Design review of the part built by this model. Coordinates are the model's own, in mm. Face numbers are marked on the shaded views. A direction names the side the tool comes from. Round coordinates to 2 decimals unless told otherwise and drop trailing zeros. Loops run counter-clockwise (first coordinate to the right, second up) from the corner with the lowest first, then second, coordinate; pieces in that order, holes last. Notation, with made-up numbers: (47.5, 45.25) - (62.5, 45.25) arc R22 ccw to (62.5, 75.25) - close; hole circle Ø3 at (48.5, 54.5). An arc over 180 degrees is marked (long way). Return JSON: item names as keys, results as strings. Group by question number.
(1) Wall thickness on L1, parallel to Y at x = -15.5, z = -20.85; L2, parallel to X at y = -25.75, z = 38.5; L3, parallel to Z at x = -5.5, y = 34.5: over which ranges is each line inside the solid? List them lowest first. Write a range as [from, to].
(2) We need section B-B, the plane y = 37. Write out the cut boundary in (x, z).
(3) Clearance check with flat-ended pins moving along their axes: pin 1 (1.5 mm diameter, centred on x = -6.5, z = 6, fed in from -Y); pin 2 (21.5 mm diameter, centred on x = -3, z = 15, fed in from +Y); pin 3 (6.5 mm diameter, centred on y = -36.5, z = 38.5, fed in from -X). State where each tip first meets the part, or that it passes through.
(4) We need section A-A, the plane x = -15.5. Write out the cut boundary in (y, z).
(5) For the marked faces 1, 2, 3, 4 and 5, list the 3-axis set-ups (+Z, -Z, +X, -X, +Y, -Y) from which the entire face can be reached by the end or side of a thin tool; tool diameter is ignored.
(6) We need section C-C, the plane y = 26. Write out the cut boundary in (x, z), and give its area (3 significant figures).
(7) We need section D-D, the plane z = 31.5. Write out the cut boundary in (x, y), and give its area (3 significant figures).
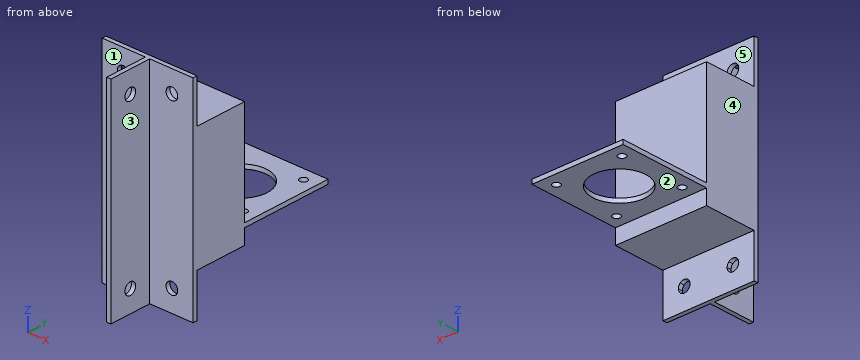
from build123d import *

# Parameters (mm, degrees)
SKETCH1_W           = 43
SKETCH1_H           = 2
BOSS_EXTRUDE1_DEPTH = 43
SKETCH1_3_W         = 43
SKETCH1_3_H         = 97
BOSS_EXTRUDE2_DEPTH = 26.5
CUT_EXTRUDE1_REACH  = 85.278
SKETCH2_R           = 12.5
SKETCH2_R_2         = 1.75
CUT_EXTRUDE2_REACH  = 70.29
SKETCH1_4_R         = 2.75
SKETCH3_W           = 43
SKETCH3_H           = 20
CUT_EXTRUDE3_DEPTH  = 24.5
SKETCH4_W           = 2
SKETCH4_H           = 97
BOSS_EXTRUDE3_DEPTH = 20
CUT_EXTRUDE4_REACH  = 72.857
SKETCH5_R           = 2.75


with BuildPart() as part:
    # Sketch1 → Boss-Extrude1 (new body)
    with BuildSketch(Plane(origin=(0, 0, 0), x_dir=(1, 0, 0), z_dir=(0, 1, 0))):
        with Locations((0, 20.5)):
            Rectangle(SKETCH1_W, SKETCH1_H)
    extrude(amount=BOSS_EXTRUDE1_DEPTH)

    # Sketch1_3 → Boss-Extrude2 (add)
    with BuildSketch(Plane(origin=(0, 0, 0), x_dir=(1, 0, 0), z_dir=(0, 1, 0))):
        Rectangle(SKETCH1_3_W, SKETCH1_3_H)
    extrude(amount=-BOSS_EXTRUDE2_DEPTH)

    # Sketch2 → Cut-Extrude1 (cut, up to next)
    with BuildSketch(Plane.XY.offset(-19.5), mode=Mode.PRIVATE) as cut_extrude1_sk1:
        with Locations((0, 21.5)):
            Circle(SKETCH2_R)
    cut_extrude1_tool1 = extrude(cut_extrude1_sk1.sketch, amount=-CUT_EXTRUDE1_REACH, mode=Mode.PRIVATE) & part.part
    # Sketch2 → Cut-Extrude1 (cut, up to next)
    with BuildSketch(Plane.XY.offset(-19.5), mode=Mode.PRIVATE) as cut_extrude1_sk2:
        with Locations((-15.5, 37)):
            Circle(SKETCH2_R_2)
    cut_extrude1_tool2 = extrude(cut_extrude1_sk2.sketch, amount=-CUT_EXTRUDE1_REACH, mode=Mode.PRIVATE) & part.part
    # Sketch2 → Cut-Extrude1 (cut, up to next)
    with BuildSketch(Plane.XY.offset(-19.5), mode=Mode.PRIVATE) as cut_extrude1_sk3:
        with Locations((15.5, 37)):
            Circle(SKETCH2_R_2)
    cut_extrude1_tool3 = extrude(cut_extrude1_sk3.sketch, amount=-CUT_EXTRUDE1_REACH, mode=Mode.PRIVATE) & part.part
    # Sketch2 → Cut-Extrude1 (cut, up to next)
    with BuildSketch(Plane.XY.offset(-19.5), mode=Mode.PRIVATE) as cut_extrude1_sk4:
        with Locations((15.5, 6)):
            Circle(SKETCH2_R_2)
    cut_extrude1_tool4 = extrude(cut_extrude1_sk4.sketch, amount=-CUT_EXTRUDE1_REACH, mode=Mode.PRIVATE) & part.part
    # Sketch2 → Cut-Extrude1 (cut, up to next)
    with BuildSketch(Plane.XY.offset(-19.5), mode=Mode.PRIVATE) as cut_extrude1_sk5:
        with Locations((-15.5, 6)):
            Circle(SKETCH2_R_2)
    cut_extrude1_tool5 = extrude(cut_extrude1_sk5.sketch, amount=-CUT_EXTRUDE1_REACH, mode=Mode.PRIVATE) & part.part
    add(cut_extrude1_tool1.solids().sort_by_distance((0, 21.5, -19.5))[0], mode=Mode.SUBTRACT)
    add(cut_extrude1_tool2.solids().sort_by_distance((-15.5, 37, -19.5))[0], mode=Mode.SUBTRACT)
    add(cut_extrude1_tool3.solids().sort_by_distance((15.5, 37, -19.5))[0], mode=Mode.SUBTRACT)
    add(cut_extrude1_tool4.solids().sort_by_distance((15.5, 6, -19.5))[0], mode=Mode.SUBTRACT)
    add(cut_extrude1_tool5.solids().sort_by_distance((-15.5, 6, -19.5))[0], mode=Mode.SUBTRACT)

    # Sketch1_4 → Cut-Extrude2 (cut, up to next)
    with BuildSketch(Plane(origin=(0, 0, 0), x_dir=(1, 0, 0), z_dir=(0, 1, 0)), mode=Mode.PRIVATE) as cut_extrude2_sk1:
        with Locations(Location((-11.5, -38.5, 0), (0, 0, 270))):
            Circle(SKETCH1_4_R)
    cut_extrude2_tool1 = extrude(cut_extrude2_sk1.sketch, amount=-CUT_EXTRUDE2_REACH, mode=Mode.PRIVATE) & part.part
    # Sketch1_4 → Cut-Extrude2 (cut, up to next)
    with BuildSketch(Plane(origin=(0, 0, 0), x_dir=(1, 0, 0), z_dir=(0, 1, 0)), mode=Mode.PRIVATE) as cut_extrude2_sk2:
        with Locations(Location((11.5, -38.5, 0), (0, 0, 270))):
            Circle(SKETCH1_4_R)
    cut_extrude2_tool2 = extrude(cut_extrude2_sk2.sketch, amount=-CUT_EXTRUDE2_REACH, mode=Mode.PRIVATE) & part.part
    # Sketch1_4 → Cut-Extrude2 (cut, up to next)
    with BuildSketch(Plane(origin=(0, 0, 0), x_dir=(1, 0, 0), z_dir=(0, 1, 0)), mode=Mode.PRIVATE) as cut_extrude2_sk3:
        with BuildLine():
            ThreePointArc((-8.75, 38.5), (-12.589033706, 41.025174368), (-13.387458609, 36.5))
            Line((-13.387458609, 36.5), (-9.612541391, 36.5))
            ThreePointArc((-9.612541391, 36.5), (-8.974825632, 37.410966294), (-8.75, 38.5))
        make_face()
    cut_extrude2_tool3 = extrude(cut_extrude2_sk3.sketch, amount=-CUT_EXTRUDE2_REACH, mode=Mode.PRIVATE) & part.part
    # Sketch1_4 → Cut-Extrude2 (cut, up to next)
    with BuildSketch(Plane(origin=(0, 0, 0), x_dir=(1, 0, 0), z_dir=(0, 1, 0)), mode=Mode.PRIVATE) as cut_extrude2_sk4:
        with BuildLine():
            Line((-9.612541391, 36.5), (-13.387458609, 36.5))
            ThreePointArc((-13.387458609, 36.5), (-11.5, 35.75), (-9.612541391, 36.5))
        make_face()
    cut_extrude2_tool4 = extrude(cut_extrude2_sk4.sketch, amount=-CUT_EXTRUDE2_REACH, mode=Mode.PRIVATE) & part.part
    # Sketch1_4 → Cut-Extrude2 (cut, up to next)
    with BuildSketch(Plane(origin=(0, 0, 0), x_dir=(1, 0, 0), z_dir=(0, 1, 0)), mode=Mode.PRIVATE) as cut_extrude2_sk5:
        with BuildLine():
            ThreePointArc((9.612541391, 36.5), (11.5, 35.75), (13.387458609, 36.5))
            Line((13.387458609, 36.5), (9.612541391, 36.5))
        make_face()
    cut_extrude2_tool5 = extrude(cut_extrude2_sk5.sketch, amount=-CUT_EXTRUDE2_REACH, mode=Mode.PRIVATE) & part.part
    # Sketch1_4 → Cut-Extrude2 (cut, up to next)
    with BuildSketch(Plane(origin=(0, 0, 0), x_dir=(1, 0, 0), z_dir=(0, 1, 0)), mode=Mode.PRIVATE) as cut_extrude2_sk6:
        with BuildLine():
            Line((9.612541391, 36.5), (13.387458609, 36.5))
            ThreePointArc((13.387458609, 36.5), (14.025174368, 37.410966294), (14.25, 38.5))
            ThreePointArc((14.25, 38.5), (10.410966294, 41.025174368), (9.612541391, 36.5))
        make_face()
    cut_extrude2_tool6 = extrude(cut_extrude2_sk6.sketch, amount=-CUT_EXTRUDE2_REACH, mode=Mode.PRIVATE) & part.part
    # Sketch1_4 → Cut-Extrude2 (cut, up to next)
    with BuildSketch(Plane(origin=(0, 0, 0), x_dir=(1, 0, 0), z_dir=(0, 1, 0)), mode=Mode.PRIVATE) as cut_extrude2_sk7:
        with BuildLine():
            ThreePointArc((9.612541391, 36.5), (11.5, 35.75), (13.387458609, 36.5))
            Line((13.387458609, 36.5), (9.612541391, 36.5))
        make_face()
    cut_extrude2_tool7 = extrude(cut_extrude2_sk7.sketch, amount=-CUT_EXTRUDE2_REACH, mode=Mode.PRIVATE) & part.part
    # Sketch1_4 → Cut-Extrude2 (cut, up to next)
    with BuildSketch(Plane(origin=(0, 0, 0), x_dir=(1, 0, 0), z_dir=(0, 1, 0)), mode=Mode.PRIVATE) as cut_extrude2_sk8:
        with BuildLine():
            Line((9.612541391, 36.5), (13.387458609, 36.5))
            ThreePointArc((13.387458609, 36.5), (14.025174368, 37.410966294), (14.25, 38.5))
            ThreePointArc((14.25, 38.5), (10.410966294, 41.025174368), (9.612541391, 36.5))
        make_face()
    cut_extrude2_tool8 = extrude(cut_extrude2_sk8.sketch, amount=-CUT_EXTRUDE2_REACH, mode=Mode.PRIVATE) & part.part
    # Sketch1_4 → Cut-Extrude2 (cut, up to next)
    with BuildSketch(Plane(origin=(0, 0, 0), x_dir=(1, 0, 0), z_dir=(0, 1, 0)), mode=Mode.PRIVATE) as cut_extrude2_sk9:
        with BuildLine():
            ThreePointArc((-8.75, 38.5), (-12.589033706, 41.025174368), (-13.387458609, 36.5))
            Line((-13.387458609, 36.5), (-9.612541391, 36.5))
            ThreePointArc((-9.612541391, 36.5), (-8.974825632, 37.410966294), (-8.75, 38.5))
        make_face()
    cut_extrude2_tool9 = extrude(cut_extrude2_sk9.sketch, amount=-CUT_EXTRUDE2_REACH, mode=Mode.PRIVATE) & part.part
    # Sketch1_4 → Cut-Extrude2 (cut, up to next)
    with BuildSketch(Plane(origin=(0, 0, 0), x_dir=(1, 0, 0), z_dir=(0, 1, 0)), mode=Mode.PRIVATE) as cut_extrude2_sk10:
        with BuildLine():
            Line((-9.612541391, 36.5), (-13.387458609, 36.5))
            ThreePointArc((-13.387458609, 36.5), (-11.5, 35.75), (-9.612541391, 36.5))
        make_face()
    cut_extrude2_tool10 = extrude(cut_extrude2_sk10.sketch, amount=-CUT_EXTRUDE2_REACH, mode=Mode.PRIVATE) & part.part
    add(cut_extrude2_tool1.solids().sort_by_distance((-11.5, 0, 38.5))[0], mode=Mode.SUBTRACT)
    add(cut_extrude2_tool2.solids().sort_by_distance((11.5, 0, 38.5))[0], mode=Mode.SUBTRACT)
    add(cut_extrude2_tool3.solids().sort_by_distance((-11.5, 0, -38.705511))[0], mode=Mode.SUBTRACT)
    add(cut_extrude2_tool4.solids().sort_by_distance((-11.5, 0, -36.196191))[0], mode=Mode.SUBTRACT)
    add(cut_extrude2_tool5.solids().sort_by_distance((11.5, 0, -36.196191))[0], mode=Mode.SUBTRACT)
    add(cut_extrude2_tool6.solids().sort_by_distance((11.5, 0, -38.705511))[0], mode=Mode.SUBTRACT)
    add(cut_extrude2_tool7.solids().sort_by_distance((11.5, 0, -36.196191))[0], mode=Mode.SUBTRACT)
    add(cut_extrude2_tool8.solids().sort_by_distance((11.5, 0, -38.705511))[0], mode=Mode.SUBTRACT)
    add(cut_extrude2_tool9.solids().sort_by_distance((-11.5, 0, -38.705511))[0], mode=Mode.SUBTRACT)
    add(cut_extrude2_tool10.solids().sort_by_distance((-11.5, 0, -36.196191))[0], mode=Mode.SUBTRACT)

    # Sketch3 → Cut-Extrude3 (cut)
    with BuildSketch(Plane(origin=(0, 0, 0), x_dir=(1, 0, 0), z_dir=(0, 1, 0))):
        with Locations((0, -38.5)):
            Rectangle(SKETCH3_W, SKETCH3_H)
        with Locations((0, 38.5)):
            Rectangle(SKETCH3_W, SKETCH3_H)
    extrude(amount=-CUT_EXTRUDE3_DEPTH, mode=Mode.SUBTRACT)

    # Sketch4 → Boss-Extrude3 (add)
    with BuildSketch(Plane.XZ.offset(26.5)):
        Rectangle(SKETCH4_W, SKETCH4_H)
    extrude(amount=BOSS_EXTRUDE3_DEPTH)

    # Sketch5 → Cut-Extrude4 (cut, up to next)
    with BuildSketch(Plane(origin=(1, 0, 0), x_dir=(0, 0, -1), z_dir=(1, 0, 0)), mode=Mode.PRIVATE) as cut_extrude4_sk1:
        with Locations((38.5, -36.5)):
            Circle(SKETCH5_R)
    cut_extrude4_tool1 = extrude(cut_extrude4_sk1.sketch, amount=-CUT_EXTRUDE4_REACH, mode=Mode.PRIVATE) & part.part
    # Sketch5 → Cut-Extrude4 (cut, up to next)
    with BuildSketch(Plane(origin=(1, 0, 0), x_dir=(0, 0, -1), z_dir=(1, 0, 0)), mode=Mode.PRIVATE) as cut_extrude4_sk2:
        with Locations((-38.5, -36.5)):
            Circle(SKETCH5_R)
    cut_extrude4_tool2 = extrude(cut_extrude4_sk2.sketch, amount=-CUT_EXTRUDE4_REACH, mode=Mode.PRIVATE) & part.part
    add(cut_extrude4_tool1.solids().sort_by_distance((1, -36.5, -38.5))[0], mode=Mode.SUBTRACT)
    add(cut_extrude4_tool2.solids().sort_by_distance((1, -36.5, 38.5))[0], mode=Mode.SUBTRACT)


solid = part.part
Solutions:
{
 "1": {"L1": "[-26.5, 4.25], [7.75, 35.25], [38.75, 43]", "L2": "[-21.5, -14.25], [-8.75, 8.75], [14.25, 21.5]", "L3": "[-21.5, -19.5]"},
 "2": {"outline": "(-21.5, -21.5) - (-17.25, -21.5) - (-17.25, -19.5) - (-21.5, -19.5) - close; (-13.75, -21.5) - (13.75, -21.5) - (13.75, -19.5) - (-13.75, -19.5) - close; (17.25, -21.5) - (21.5, -21.5) - (21.5, -19.5) - (17.25, -19.5) - close"},
 "3": {"pin 1": "y = -26.5", "pin 2": "y = 0", "pin 3": "x = -1"},
 "4": {"outline": "(-26.5, -48.5) - (-24.5, -48.5) - (-24.5, -28.5) - (0, -28.5) - (0, -21.5) - (4.25, -21.5) - (4.25, -19.5) - (0, -19.5) - (0, 28.5) - (-24.5, 28.5) - (-24.5, 48.5) - (-26.5, 48.5) - close; (7.75, -21.5) - (35.25, -21.5) - (35.25, -19.5) - (7.75, -19.5) - close; (38.75, -21.5) - (43, -21.5) - (43, -19.5) - (38.75, -19.5) - close"},
 "5": {"face 1": "+Z, -Z, -X, -Y", "face 2": "-Z, +X, -X, +Y", "face 3": "+Z, -Z, +X, -Y", "face 4": "+Z, -Z, -X, +Y, -Y", "face 5": "+Z, +X, -X, +Y"},
 "6": {"outline": "(-21.5, -21.5) - (-11.66, -21.5) - (-11.66, -19.5) - (-21.5, -19.5) - close; (11.66, -21.5) - (21.5, -21.5) - (21.5, -19.5) - (11.66, -19.5) - close", "area": "39.4 mm^2"},
 "7": {"outline": "(-21.5, -26.5) - (-1, -26.5) - (-1, -46.5) - (1, -46.5) - (1, -26.5) - (21.5, -26.5) - (21.5, -24.5) - (-21.5, -24.5) - close", "area": "126 mm^2"}
}
